Source: CAD feature listing. Evaluate the final solid. Frame: model axes, mm. Face numbers are marked on the shaded views. A direction names the side the tool comes from. Give positions to 0.01 mm unless a question says otherwise; leave off trailing zeros. Write each loop counter-clockwise with the first axis right and the second up, starting at its lowest first coordinate (ties: lowest second). Pieces come first, ordered by that corner, then holes. Notation, with made-up numbers: (86, 54) -> (130, 54) arc R12 cw to (130, 75) -> close; hole circle Ø3 at (-24, -37). An arc over 180 degrees is marked (long way). Answer as a JSON object with one key per item and string values. Group by question number.
Item 1: Section query C-C on x = 5.5. Return the cut outline in (y, z), plus the area to 3 significant figures.
Item 2: Access query for the marked faces 4 and 5. Directions: +Z, -Z, +X, -X, +Y, -Y. A direction counts if a zero-diameter tool reaches every point of the face in a straight line with its end or side. Return the directions, or none.
Item 3: First-contact query: pin 1 Ø2 at (x, y) = (4.5, 16) entering from -Z; pin 2 Ø12 at (y, z) = (11, -50) entering from +X; pin 3 Ø2 at (y, z) = (22, 6.5) entering from +X. Flat tips, straight axial feed; report the tip coordinate or a pass-through.
Item 4: Ray query, probe 1 along Z at (x, y) = (3.5, 0); probe 2 along Z at (x, y) = (4, 0); probe 3 along Y at (x, z) = (3, 19). Return the intervals inside material, ascending. Write a range as from..to.
Item 5: Pull-direction query (Y, two-part tool) for the marked faces 1, 2 and 3; classes: pulls with the +Y half, pulls with the -Y half, needs draft (parallel to the pull), parting line crosses it, or undercut.
Item 6: Section query D-D on x = 36. Return the cut outline in (y, z).
Item 7: Section query A-A on z = 0. Return the cut outline in (x, y), plus the area to 3 significant figures.
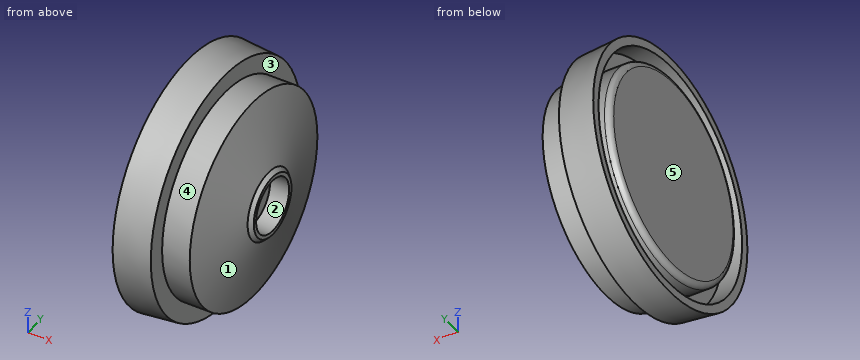
from build123d import *

# Parameters (mm, degrees)
FILLET1_R = 3


with BuildPart() as part:
    # Sketch1 → Revolve1 (revolve)
    with BuildSketch(Plane.XY):
        Polygon((0, 65.4), (19, 63.737715393), (19, 54.15), (33.5, 54.15), (41.5, 18), (43.5, 16), (43.5, 14), (33.5, 14), (33.5, 0), (0, 0), (-1.6, 0), (-1.6, 53.6), (10.4, 53.6), (10.4, 60.9), (0, 60.9), align=None)
    revolve(axis=Axis((0, 0, 0), (1, 0, 0)))

    # Fillet1
    fillet1_edges = [part.edges().sort_by_distance(p)[0] for p in [
        (-1.6, -53.6, 0),
    ]]
    fillet(fillet1_edges, radius=FILLET1_R)


solid = part.part
Worked answers:
{
 "1": {"outline": "circle Ø129.84 at (0, 0); circle Ø107.2 at (0, 0); hole circle Ø121.8 at (0, 0)", "area": "10,600 mm^2"},
 "2": {"face 4": "+X", "face 5": "+Z, -Z, -X, +Y, -Y"},
 "3": {"pin 1": "z = -63.27", "pin 2": "x = 35.48", "pin 3": "x = 40.63"},
 "4": {"probe 1": "-65.09..-60.9, -53.6..53.6, 60.9..65.09", "probe 2": "-65.05..-60.9, -53.6..53.6, 60.9..65.05", "probe 3": "-62.3..-57.86, -50.12..50.12, 57.86..62.3"},
 "5": {"face 1": "parting line crosses it", "face 2": "undercut", "face 3": "needs draft"},
 "6": {"outline": "circle Ø85.71 at (0, 0); hole circle Ø28 at (0, 0)"},
 "7": {"outline": "(-1.6, -50.6) arc R3 ccw to (1.4, -53.6) -> (10.4, -53.6) -> (10.4, -60.9) -> (0, -60.9) -> (0, -65.4) -> (19, -63.74) -> (19, -54.15) -> (33.5, -54.15) -> (41.5, -18) -> (43.5, -16) -> (43.5, -14) -> (33.5, -14) -> (33.5, 14) -> (43.5, 14) -> (43.5, 16) -> (41.5, 18) -> (33.5, 54.15) -> (19, 54.15) -> (19, 63.74) -> (0, 65.4) -> (0, 60.9) -> (10.4, 60.9) -> (10.4, 53.6) -> (1.4, 53.6) arc R3 ccw to (-1.6, 50.6) -> close", "area": "4,400 mm^2"}
}
